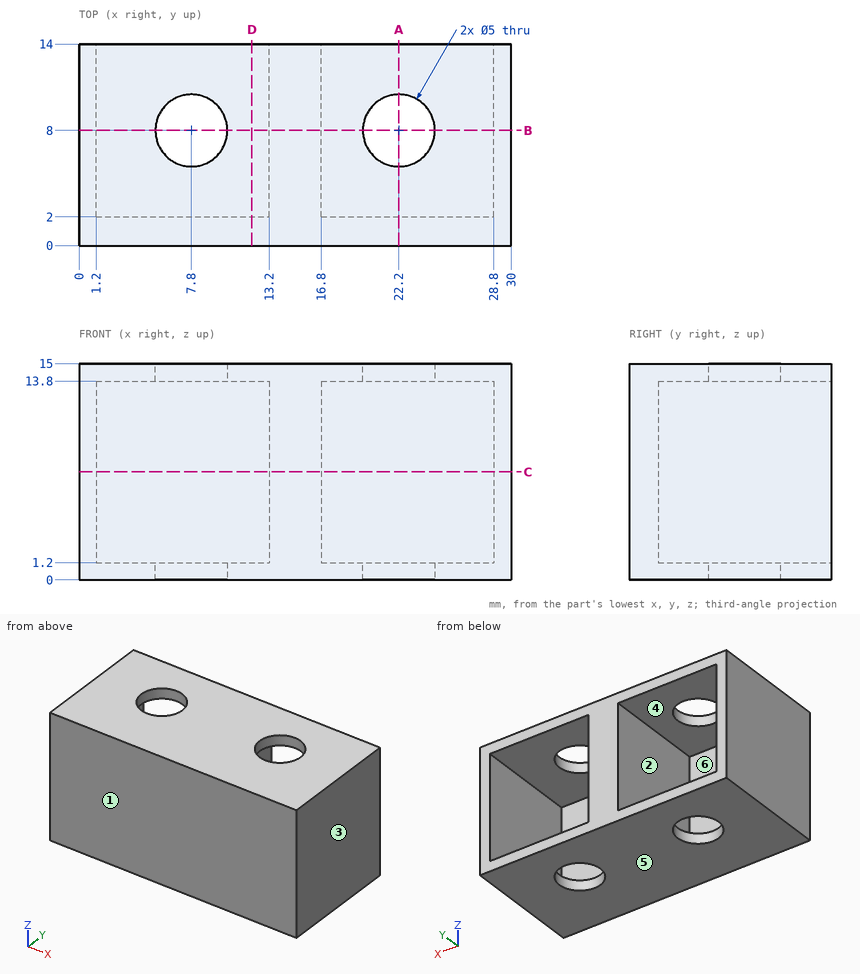
Input: dimensioned drawing with shaded views. Units: mm. Origin: part minimum x, y, z. A direction names the side the tool comes from. Give positions to 0.01 mm unless a question says otherwise; leave off trailing zeros. Write each loop counter-clockwise with the first axis right and the second up, starting at its lowest first coordinate (ties: lowest second). Pieces come first, ordered by that corner, then holes.
1. Section query A-A (x = 22.2). Return the cut outline in (y, z), then the cut area to 3 significant figures.
2. First-contact query: pin 1 (6 mm diameter, centred on x = 22, z = 9.5, fed in from +Y). Flat tip, straight axial feed; report the tip coordinate or a pass-through.
3. Section query D-D (x = 12). Return the cut outline in (y, z).
4. Access query for the marked faces 1 and 2. Directions: +Z, -Z, +X, -X, +Y, -Y. A direction counts if a zero-diameter tool reaches every point of the face in a straight line with its end or side. Return the directions, or none.
5. Material intervals for line 1 along X through (y, z) = (5, 8); line 2 along Z through (x, y) = (2, 3); line 3 along Y through (x, z) = (22.2, 0.45), sorted ascending.
6. Section query B-B (y = 8). Return the cut outline in (x, z), then the cut area to 3 significant figures.
7. Section query C-C (z = 7.5). Return the cut outline in (x, y).
8. Pull-direction query (X, two-part tool) for the marked faces 3, 4, 5 and 6; classes: +X half, -X half, draft (parallel to the pull), parting line (faces both ways), or undercut.
Output values:
1. outline: (0, 0) - (5.5, 0) - (5.5, 1.2) - (2, 1.2) - (2, 13.8) - (5.5, 13.8) - (5.5, 15) - (0, 15) - close; (10.5, 0) - (14, 0) - (14, 1.2) - (10.5, 1.2) - close; (10.5, 13.8) - (14, 13.8) - (14, 15) - (10.5, 15) - close
1. area: 46.8 mm2
2. pin 1: stops at y = 2
3. outline: (0, 0) - (14, 0) - (14, 1.2) - (2, 1.2) - (2, 13.8) - (14, 13.8) - (14, 15) - (0, 15) - close
4. face 1: +Z, -Z, +X, -X, -Y
4. face 2: +Y
5. line 1: x = 0 to 1.2, 13.2 to 16.8, 28.8 to 30
5. line 2: z = 0 to 1.2, 13.8 to 15
5. line 3: y = 0 to 5.5, 10.5 to 14
6. outline: (0, 0) - (5.3, 0) - (5.3, 1.2) - (1.2, 1.2) - (1.2, 13.8) - (5.3, 13.8) - (5.3, 15) - (0, 15) - close; (10.3, 0) - (19.7, 0) - (19.7, 1.2) - (16.8, 1.2) - (16.8, 13.8) - (19.7, 13.8) - (19.7, 15) - (10.3, 15) - (10.3, 13.8) - (13.2, 13.8) - (13.2, 1.2) - (10.3, 1.2) - close; (24.7, 0) - (30, 0) - (30, 15) - (24.7, 15) - (24.7, 13.8) - (28.8, 13.8) - (28.8, 1.2) - (24.7, 1.2) - close
6. area: 124 mm2
7. outline: (0, 0) - (30, 0) - (30, 14) - (28.8, 14) - (28.8, 2) - (16.8, 2) - (16.8, 14) - (13.2, 14) - (13.2, 2) - (1.2, 2) - (1.2, 14) - (0, 14) - close
8. face 3: +X half
8. face 4: undercut
8. face 5: draft
8. face 6: undercut
